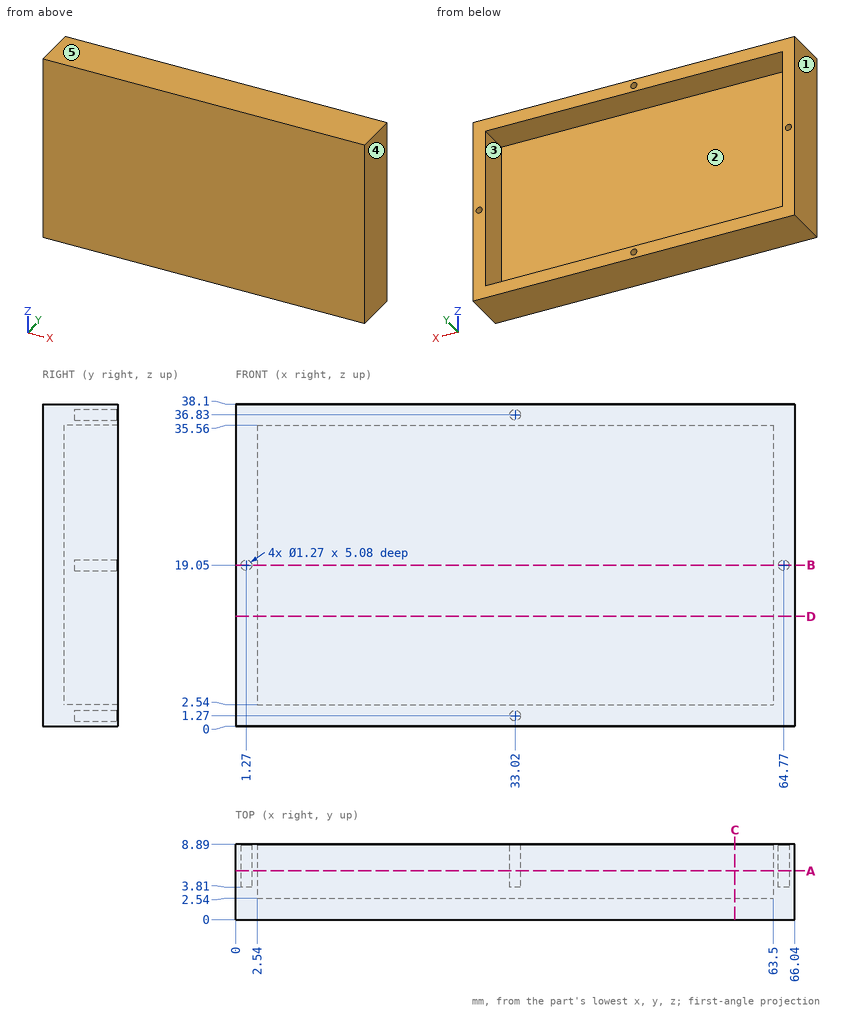
Check sheet for the drawn part. Datum: minimum x, y, z corner. Units: mm. A direction names the side the tool comes from. Round coordinates to 2 decimals unless told otherwise and drop trailing zeros. Order: outer loops, then holes, each group sorted by start corner. A loop starts at its lowest first (then second) coordinate and runs counter-clockwise, first axis right, second up. Notation, with made-up numbers: (62, 9) - (69, 9) arc R22 cw to (69, 18) - close; hole circle Ø1 at (68, 38.5). An arc over 180 degrees is marked (long way). Use a Markdown table: item, result. Add a question column.
(1) Material ranges on line 1 along X through (y, z) = (5.25, 14.5); line 2 along Z through (x, y) = (12.5, 4.5); line 3 along Z through (x, y) = (1.27, 5.4) (3 decimals), recorded low to high. Write a range as [from, to].
(2) Sectioned sample at D-D, the plane z = 13. Enter the section's corners in (x, y).
(3) Sectioned sample at C-C, the plane x = 59. Enter the section's corners in (y, z).
(4) Depth check by flat-ended pin: pin 1 (1 mm diameter, centred on x = 33.02, z = 1.27, fed in from +Y); pin 2 (10 mm diameter, centred on x = 41.5, z = 27, fed in from +Y). Enter the tip coordinate at first touch or a pass-through.
(5) Release check for a two-part mould opening along Z. For the marked faces 3, 4 and 5 record: pulls with the +Z half, pulls with the -Z half, needs draft (parallel to the pull), parting line crosses it, or undercut.
(6) Sectioned sample at A-A, the plane y = 5.75. Enter the section's corners in (x, z) (3 decimals), and give its area (3 significant figures).
(7) Tool access check on the marked faces 1 and 2. Record the directions out of +Z, -Z, +X, -X, +Y, -Y that give a thin tool (end or side, any length) a straight path to the whole face; none if there is none.
(8) Sectioned sample at B-B, the plane z = 19.05. Enter the section's corners in (x, y) (3 decimals), and give its area (3 significant figures).
Answers below:
| question | item | result |
|---|---|---|
| 1 | line 1 | [0, 2.54], [63.5, 66.04] |
| 1 | line 2 | [0, 2.54], [35.56, 38.1] |
| 1 | line 3 | [0, 18.415], [19.685, 38.1] |
| 2 | outline | (0, 0) - (66.04, 0) - (66.04, 8.89) - (63.5, 8.89) - (63.5, 2.54) - (2.54, 2.54) - (2.54, 8.89) - (0, 8.89) - close |
| 3 | outline | (0, 0) - (8.89, 0) - (8.89, 2.54) - (2.54, 2.54) - (2.54, 35.56) - (8.89, 35.56) - (8.89, 38.1) - (0, 38.1) - close |
| 4 | pin 1 | y = 3.81 |
| 4 | pin 2 | y = 2.54 |
| 5 | face 3 | undercut |
| 5 | face 4 | needs draft |
| 5 | face 5 | pulls with the +Z half |
| 6 | outline | (0, 0) - (66.04, 0) - (66.04, 38.1) - (0, 38.1) - close; hole circle Ø1.27 at (1.27, 19.05); hole (2.54, 2.54) - (63.5, 2.54) - (63.5, 35.56) - (2.54, 35.56) - close; hole circle Ø1.27 at (33.02, 1.27); hole circle Ø1.27 at (33.02, 36.83); hole circle Ø1.27 at (64.77, 19.05) |
| 6 | area | 498 mm² |
| 7 | face 1 | +Z, -Z, -X, +Y, -Y |
| 7 | face 2 | +Y |
| 8 | outline | (0, 0) - (66.04, 0) - (66.04, 8.89) - (65.405, 8.89) - (65.405, 3.81) - (64.135, 3.81) - (64.135, 8.89) - (63.5, 8.89) - (63.5, 2.54) - (2.54, 2.54) - (2.54, 8.89) - (1.905, 8.89) - (1.905, 3.81) - (0.635, 3.81) - (0.635, 8.89) - (0, 8.89) - close |
| 8 | area | 187 mm² |
